from build123d import *

# Parameters (mm, degrees)
CUT_EXTRUDE_1_DEPTH = 2


with BuildPart() as part:
    # 草图1 → 旋转1 (revolve)
    with BuildSketch(Plane.XY):
        Polygon((0, 20), (-3, 20), (-1.25, 18.25), (-1.25, 17.25), (-1.5, 17.25), (-1.5, 0), (0, 0), align=None)
    revolve(axis=Axis((0, 0, 0), (0, 1, 0)))

    # 草图2 → 切除-拉伸1 (cut)
    with BuildSketch(Plane(origin=(0, 20, 0), x_dir=(1, 0, 0), z_dir=(0, 1, 0))):
        Polygon((0.577350269, 1), (-0.577350269, 1), (-1.154700538, 0), (-0.577350269, -1), (0.577350269, -1), (1.154700538, 0), align=None)
    extrude(amount=-CUT_EXTRUDE_1_DEPTH, mode=Mode.SUBTRACT)


solid = part.part
Verification items for the finished model (mm, model axes). A direction names the side the tool comes from. Give positions to 0.01 mm unless a question says otherwise; leave off trailing zeros. Loops run counter-clockwise (first coordinate to the right, second up) from the corner with the lowest first, then second, coordinate; pieces in that order, holes last.
1) Draft check along Y on faces 4 (the flat face through (0.86, 19.01, 0.51)), 5 (the cylindrical face through (0.27, 17.74, -1.22)), 6 (the flat face through (0, 0, 0)). Enter one of: pulls with the +Y half, pulls with the -Y half, needs draft (parallel to the pull), parting line crosses it, or undercut.
2) Sectioned sample at B-B, the plane y = 6. Enter the section's corners in (x, z).
3) Set-up check for faces 1 (the cylindrical face through (1.5, 8.5, 0.07)), 2 (the flat face through (0, 20, -1.3)), 3 (the flat face through (-0.87, 19.01, 0.49)): record each of +Z, -Z, +X, -X, +Y, -Y from which the full face is reachable in a straight line by a thin tool's end or side.
4) Thickness scan on line 1 along X through (y, z) = (12.5, 0.1); line 2 along Y through (x, z) = (-0.3, 1.85); line 3 along Y through (x, z) = (-1.1, -1.4). Record the ranges inside material, lowest first.
5) Depth check by flat-ended pin: pin 1 Ø1.5 at (x, y) = (-2, 7.5) entering from +Z; pin 2 Ø3 at (y, z) = (8, 1.5) entering from -X; pin 3 Ø0.6 at (x, y) = (-0.5, 19) entering from +Z. Enter the tip coordinate at first touch or a pass-through.
6) Sectioned sample at A-A, the plane x = 0. Enter the section's corners in (y, z).
Answers:
1. face 4: needs draft
1. face 5: undercut
1. face 6: pulls with the -Y half
2. outline: circle Ø3 at (0, 0)
3. face 1: -Y
3. face 2: +Z, -Z, +X, -X, +Y
3. face 3: +Y
4. line 1: x = -1.5 to 1.5
4. line 2: y = 18.87 to 20
4. line 3: y = 18.78 to 20
5. pin 1: stops at z = 0.83
5. pin 2: stops at x = -1.5
5. pin 3: stops at z = 2.25
6. outline: (0, -1.5) - (17.25, -1.5) - (17.25, -1.25) - (18.25, -1.25) - (20, -3) - (20, -1) - (18, -1) - (18, 1) - (20, 1) - (20, 3) - (18.25, 1.25) - (17.25, 1.25) - (17.25, 1.5) - (0, 1.5) - close
